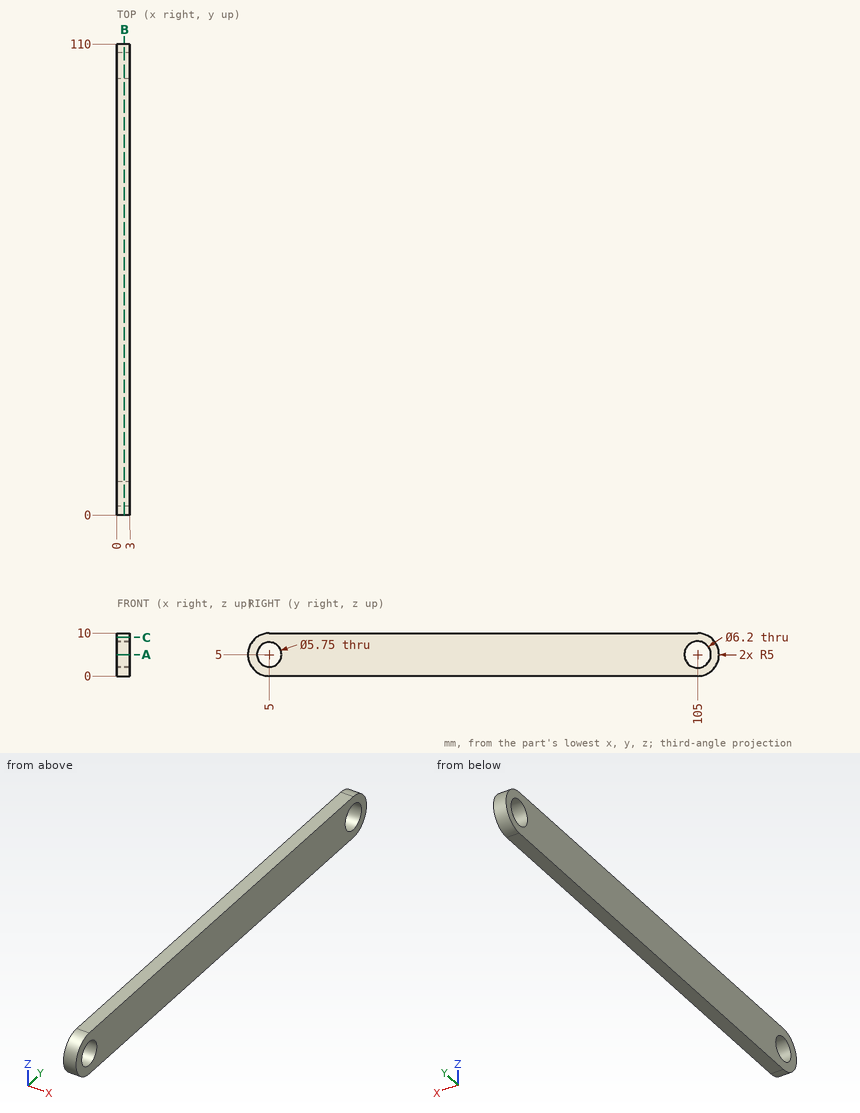
Here's the drawing with two shaded views (mm, measured from the low corner). I have some questions. Round coordinates to 2 decimals unless told otherwise and drop trailing zeros. Loops run counter-clockwise (first coordinate to the right, second up) from the corner with the lowest first, then second, coordinate; pieces in that order, holes last. Notation, with made-up numbers: (2, 65.25) -> (25, 65.25) arc R21 ccw to (25, 96.25) -> close; hole circle Ø6 at (27.25, 7.25). An arc over 180 degrees is marked (long way). Answer as CSV lines item,"result". Start each with the question number.
1. Imagine slicing it at A-A on z = 5. Write out the boundary of the cut face in (x, y) (3 decimals).
2. I need wall thicknesses on probe 1 along Y at (x, z) = (2.25, 5.25); probe 2 along Z at (x, y) = (1.5, 105); probe 3 along Z at (x, y) = (1.5, 5) (3 decimals). Which ranges of each line are inside material? Lowest first, please. Write a range as from..to.
3. Imagine slicing it at C-C on z = 9. Write out the boundary of the cut face in (x, y).
4. Imagine slicing it at B-B on x = 1.75. Write out the boundary of the cut face in (y, z) (3 decimals).
5. I'm going to push flat-ended pins straight in: P1, Ø1, axis at y = 38, z = 8.5, coming from the -X side; P2, Ø1.5, axis at x = 0.5, z = 2, coming from the +Y side. Where does each tip first touch, or does it pass through?
Solution:
1,outline,"(0, 0) -> (3, 0) -> (3, 2.125) -> (0, 2.125) -> close; (0, 7.875) -> (3, 7.875) -> (3, 101.9) -> (0, 101.9) -> close; (0, 108.1) -> (3, 108.1) -> (3, 110) -> (0, 110) -> close"
2,probe 1,"0.01..2.14, 7.86..101.91, 108.09..109.99"
2,probe 2,"0..1.9, 8.1..10"
2,probe 3,"0..2.125, 7.875..10"
3,outline,"(0, 2) -> (3, 2) -> (3, 108) -> (0, 108) -> close"
4,outline,"(5, 0) -> (105, 0) arc R5 ccw to (105, 10) -> (5, 10) arc R5 ccw to start; hole circle Ø5.75 at (5, 5); hole circle Ø6.2 at (105, 5)"
5,P1,"x = 0"
5,P2,"y = 109.47"
